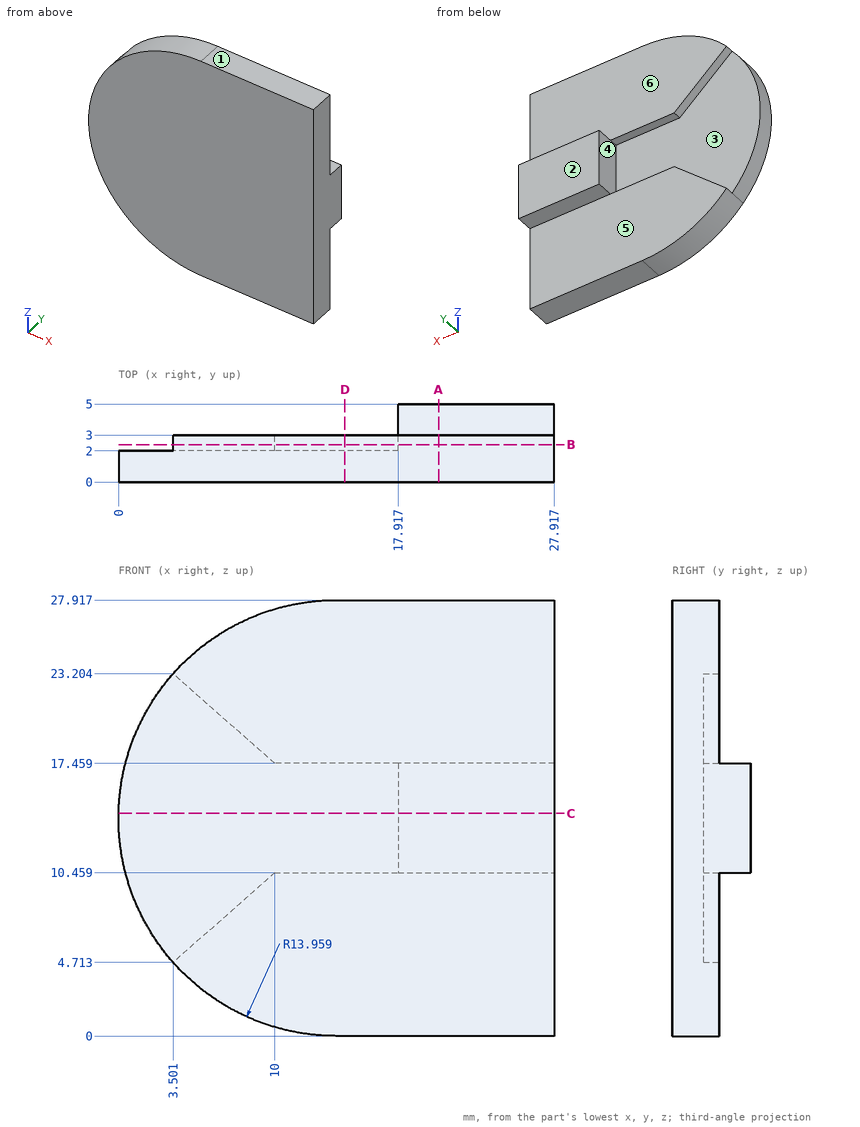
Study the drawing (mm; zero at the part's minimum x, y, z) and answer. A direction names the side the tool comes from. Give positions to 0.01 mm unless a question says otherwise; leave off trailing zeros. Write each loop counter-clockwise with the first axis right and the second up, starting at its lowest first coordinate (ties: lowest second). Pieces come first, ordered by that corner, then holes.
(1) The part is cut by section C-C on z = 14.25. Write down the section's boundary in (x, y).
Final values:
outline: (0, 0) - (27.92, 0) - (27.92, 5) - (17.92, 5) - (17.92, 2) - (0, 2) - close
(2) The part is cut by section B-B on y = 2.4. Write down the section's boundary in (x, z) (1 decimal), plus the area to 3 significant figures.
Final values:
outline: (3.5, 4.7) arc R14 ccw to (14, 0) - (27.9, 0) - (27.9, 27.9) - (14, 27.9) arc R14 ccw to (3.5, 23.2) - (10, 17.5) - (17.9, 17.5) - (17.9, 10.5) - (10, 10.5) - close
area: 513 mm2
(3) The part is cut by section D-D on x = 14.5. Write down the section's boundary in (y, z).
Final values:
outline: (0, 0) - (3, 0) - (3, 10.46) - (2, 10.46) - (2, 17.46) - (3, 17.46) - (3, 27.92) - (0, 27.92) - close
(4) The part is cut by section A-A on x = 20.5. Write down the section's boundary in (y, z).
Final values:
outline: (0, 0) - (3, 0) - (3, 10.46) - (5, 10.46) - (5, 17.46) - (3, 17.46) - (3, 27.92) - (0, 27.92) - close
(5) Which of the six approach directions +Z, -Z, +X, -X, +Y, -Y give full straight-line access (tool end or side, diameter ignored) to the marked faces 4, 5 and 6?
Final values:
face 4: -X, +Y
face 5: -Z, +X, -X, +Y
face 6: +Z, +X, -X, +Y
(6) Straight lines are drawn through the part: line 1 (Y direction, x = 20.5, z = 9.75); line 2 (X direction, y = 3.3, z = 12.75); line 3 (Y direction, x = 14.5, z = 12). For each, find the intervals that lie inside material, in ascending order.
Final values:
line 1: y = 0 to 3
line 2: x = 17.92 to 27.92
line 3: y = 0 to 2
(7) Flat-ended cylindrical pins translate along their axes: pin 1 Ø1 at (y, z) = (2.5, 23.5) entering from -X; pin 2 Ø3 at (x, z) = (13.5, 21.5) entering from +Y; pin 3 Ø1.6 at (x, y) = (25, 4) entering from -Z. Find the tip coordinate at first contact, or state that the pin passes through.
Final values:
pin 1: stops at x = 3.5
pin 2: stops at y = 3
pin 3: stops at z = 10.46
(8) The mould has two halves that part along Z. Classify the marked faces 1, 2 and 3: pulls with the +Z half, pulls with the -Z half, needs draft (parallel to the pull), parting line crosses it, or undercut.
Final values:
face 1: pulls with the +Z half
face 2: needs draft
face 3: undercut
